Drawing for the job (mm, zero at the part's lowest x, y, z). A direction names the side the tool comes from. Coordinates: 2 decimals unless noted, no trailing zeros. Write each loop counter-clockwise with the first axis right and the second up, starting at its lowest first coordinate (ties: lowest second). Pieces come first, ordered by that corner, then holes. Notation, with made-up numbers: M -3.75,53.25 L 44.25,53.25 A11 ccw 44.25,62.25 Z; hole C -23.5,49.25 d10. An arc over 180 degrees is marked long. Put each result on its own line as item: value. Start each with the question number.
Q1. Which spindle directions (+Z, -Z, +X, -X, +Y, -Y) get a long thin tool onto all of the face, cutting with end or side? Do the marked faces 1 and 2. Say none if no direction does.
Q2. Drop flat-ended pins along their axis: pin 1 (3 mm diameter, centred on y = 9.5, z = 5.5, fed in from -X); pin 2 (2 mm diameter, centred on x = 30, z = 6, fed in from -Y); pin 3 (4 mm diameter, centred on x = 59, y = 8, fed in from +Z); pin 4 (2 mm diameter, centred on x = 10, z = 3.5, fed in from -Y) (1 decimal). Give the stop position or say it passes through.
Q3. Drill centre lines: line 1 along Z through (x, y) = (31, 3.75) (1 decimal); line 2 along Y through (x, z) = (60, 9.5) (1 decimal); line 3 along Y through (x, z) = (14.5, 6.5). Where is each one in solid material? Low to high.
Q4. Cut at B-B (x = 39). Write the cut outline in (y, z), then the cut area to 3 significant figures.
Q5. Cut at A-A (x = 30.5). Write the cut outline in (y, z) (1 decimal).
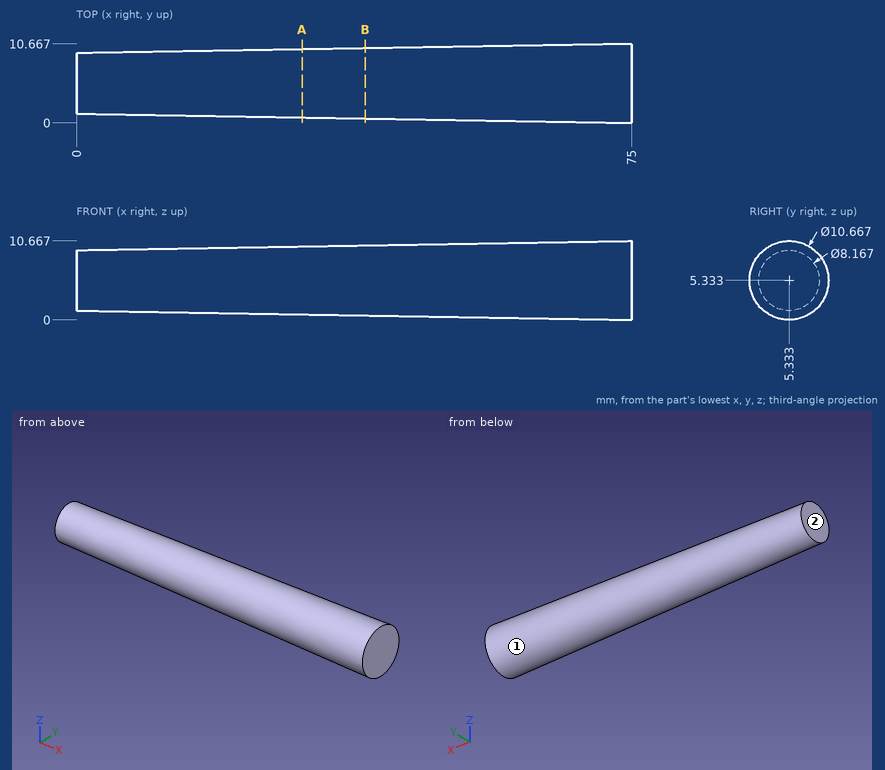
Computed values:
1. face 1: -X
1. face 2: +Z, -Z, -X, +Y, -Y
2. pin 1: x = 0
2. pin 2: y = 0.74
2. pin 3: z = 10.36
2. pin 4: y = 1.2
3. line 1: 1 to 9.7
3. line 2: 2.4 to 8.2
3. line 3: 1.17 to 9.5
4. outline: C 5.33,5.33 d9.47
4. area: 70.4 mm2
5. outline: C 5.3,5.3 d9.2
